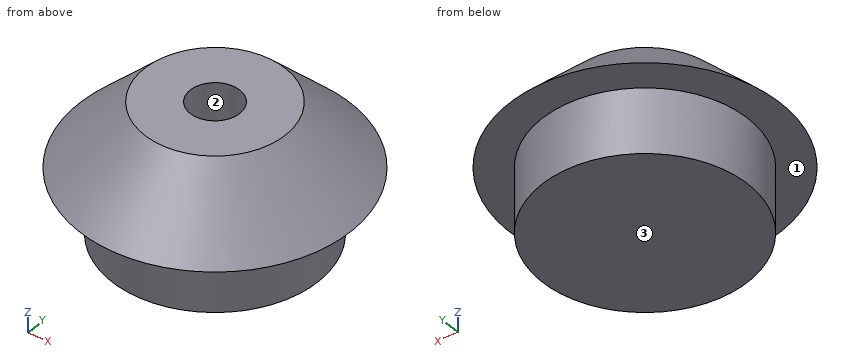
Autodesk Inventor part; units mm, degrees
ref_plane "Work Plane1" through (0, 6.0289, -1.5641) normal (0, 1, 0) x (-1, 0, 0)
ref_plane "YZ Plane" through (0, 0, 0) normal (1, 0, 0) x (0, 1, 0)
ref_plane "XY Plane" through (0, 0, 0) normal (0, 0, 1) x (1, 0, 0)
sketch "Sketch1" plane through (0, 0, 0) normal (1, 0, 0) x (0, 1, 0)
  line L0 (0.0289, 5.9359) -> (3.5289, 5.9359)
  line L1 (-1.8711, 5.9359) -> (-1.8711, -4.0641) construction
  line L2 (6.0289, 0.9359) -> (8.5289, 0.9359)
  line L3 (3.5289, 5.9359) -> (8.5289, 0.9359)
  line L4 (0.0289, -4.0641) -> (6.0289, -4.0641)
  line L5 (6.0289, -4.0641) -> (6.0289, 0.9359)
  line L6 (0.0289, 5.9359) -> (0.0289, -0.0641)
  line L7 (0.0289, -0.0641) -> (-1.8711, -0.0641)
  line L8 (-1.8711, -4.0641) -> (0.0289, -4.0641)
  line L9 (-1.8711, -0.0641) -> (-1.8711, -4.0641)
  point P0 (0, 0)
  dimension "d0" = 3.5
  dimension "d3" = 10
  dimension "d11" = 6
revolve "Revolution1" add sketch "Sketch1" angle 360 about axis through (0, -1.8711, 5.9359) along (0, 0, -1)
ref_plane "Work Plane1" through (0, 6.0289, -1.5641) normal (0, 1, 0) x (-1, 0, 0)
properties part number "guide"
Geometry check sheet. Reference: the model listing, model coordinates, mm. Face numbers are marked on the shaded views. A direction names the side the tool comes from. Coordinates: 2 decimals unless noted, no trailing zeros. Order: outer loops, then holes, each group sorted by start corner. A loop starts at its lowest first (then second) coordinate and runs counter-clockwise, first axis right, second up.
Item 1: Depth check by flat-ended pin: pin 1 (4 mm diameter, centred on x = 6.5, z = 3, fed in from -Y); pin 2 (1.9 mm diameter, centred on x = -0.5, y = -2.5, fed in from +Z); pin 3 (1 mm diameter, centred on y = -8, z = 1, fed in from +X). Enter the tip coordinate at first touch or a pass-through.
Item 2: Section check C-C (z = 2.5). Enter the section's corners in (x, y), plus the area to 3 significant figures.
Item 3: Section check D-D (z = 1.25). Enter the section's corners in (x, y), plus the area to 3 significant figures.
Item 4: Section check B-B (z = -3.5). Enter the section's corners in (x, y), plus the area to 3 significant figures.
Item 5: Section check A-A (x = 0). Enter the section's corners in (y, z).
Item 6: Tool access check on the marked faces 1, 2 and 3. Record the directions out of +Z, -Z, +X, -X, +Y, -Y that give a thin tool (end or side, any length) a straight path to the whole face; none if there is none.
Item 7: Scan lines: line 1 along X through (y, z) = (-0.5, 1.25); line 2 along Y through (x, z) = (5.75, -0.25); line 3 along X through (y, z) = (-1.75, -1.75). Record each from-to range of solid material in increasing order.
Check sheet entries:
1. pin 1: stops at y = -10.3
1. pin 2: stops at z = -0.06
1. pin 3: stops at x = 8.74
2. outline: circle Ø17.67 at (0, -1.87); hole circle Ø3.8 at (0, -1.87)
2. area: 234 mm2
3. outline: circle Ø20.17 at (0, -1.87); hole circle Ø3.8 at (0, -1.87)
3. area: 308 mm2
4. outline: circle Ø15.8 at (0, -1.87)
4. area: 196 mm2
5. outline: (-12.27, 0.94) - (-9.77, 0.94) - (-9.77, -4.06) - (6.03, -4.06) - (6.03, 0.94) - (8.53, 0.94) - (3.53, 5.94) - (0.03, 5.94) - (0.03, -0.06) - (-3.77, -0.06) - (-3.77, 5.94) - (-7.27, 5.94) - close
6. face 1: -Z
6. face 2: +Z
6. face 3: -Z, +X, -X, +Y, -Y
7. line 1: x = -9.99 to -1.32, 1.32 to 9.99
7. line 2: y = -7.29 to 3.55
7. line 3: x = -7.9 to 7.9
